Check sheet for the drawn part. Datum: minimum x, y, z corner. Units: mm. A direction names the side the tool comes from. Give positions to 0.01 mm unless a question says otherwise; leave off trailing zeros. Order: outer loops, then holes, each group sorted by start corner. A loop starts at its lowest first (then second) coordinate and runs counter-clockwise, first axis right, second up. Notation, with made-up numbers: M -19,46 L 11,46 A13 ccw 11,55 Z; hole C 81.25,84 d5. An arc over 180 degrees is marked long. Put each result on its own line as item: value. Start each with the question number.
Q1. Section check B-B on x = 10.75. Record the cut outline in (y, z).
Q2. Section check D-D on z = 10.5. Record the cut outline in (x, y).
Q3. Section check C-C on z = 19. Record the cut outline in (x, y).
Q4. Material ranges on L1, parallel to Y at x = 13, z = 8.5; L2, parallel to Y at x = 16, z = 21.25; L3, parallel to X at y = 4.5, z = 17.75, recorded low to high.
Q5. Section check A-A on y = 13. Record the cut outline in (x, z), then the cut area to 3 significant figures.
Q6. Go/stop test with flat-tipped pins: pin 1 (4 mm diameter, centred on y = 20, z = 19, fed in from -X); pin 2 (10 mm diameter, centred on y = 18.5, z = 13.5, fed in from +X); pin 3 (7 mm diameter, centred on x = 13, y = 13, fed in from -Z); pin 4 (1.5 mm diameter, centred on x = 4, z = 21.5, fed in from -Y). Record where each tip stops, or that it passes through.
Q7. Access from +Z, -Z, +X, -X, +Y, -Y to the whole of each face (thin tool, end or side, straight path). Record for the marked faces 1, 2 and 3.
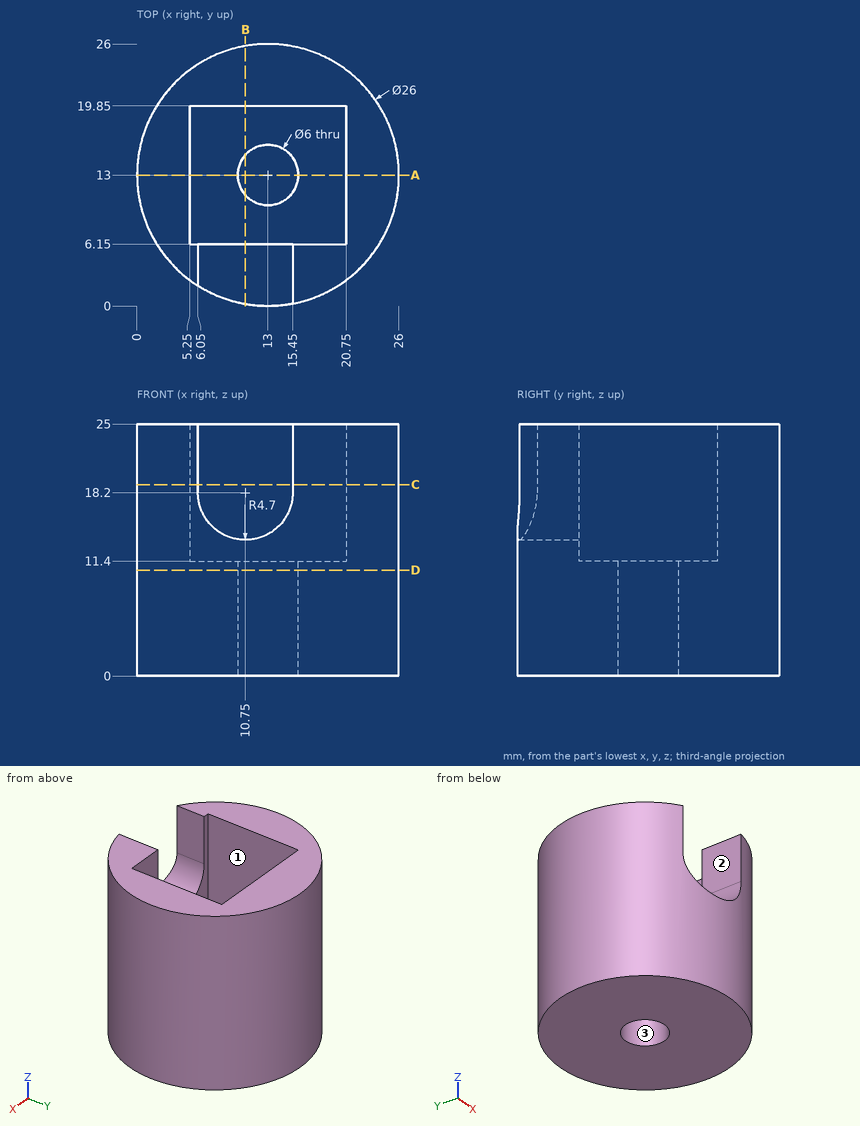
Results found:
1. outline: M 0.2,0 L 11.02,0 L 11.02,11.4 L 6.15,11.4 L 6.15,13.5 L 0.2,13.5 Z; M 14.98,0 L 25.8,0 L 25.8,25 L 19.85,25 L 19.85,11.4 L 14.98,11.4 Z
2. outline: C 13,13 d26; hole C 13,13 d6
3. outline: M 5.25,6.15 L 5.25,19.85 L 20.75,19.85 L 20.75,6.15 L 15.45,6.15 L 15.45,0.23 A13 ccw long 6.05,2.01 L 6.05,6.15 Z
4. L1: y = 0 to 10, 16 to 26
4. L2: y = 0.35 to 6.15, 19.85 to 25.65
4. L3: x = 3.16 to 6.07, 15.43 to 22.84
5. outline: M 0,0 L 10,0 L 10,11.4 L 5.25,11.4 L 5.25,25 L 0,25 Z; M 16,0 L 26,0 L 26,25 L 20.75,25 L 20.75,11.4 L 16,11.4 Z
5. area: 371 mm^2
6. pin 1: stops at x = 1
6. pin 2: stops at x = 25.99
6. pin 3: stops at z = 0
6. pin 4: stops at y = 2.95
7. face 1: +Z
7. face 2: +Z, -Y
7. face 3: +Z, -Z
